Source: CAD feature listing. Evaluate the final solid. Frame: model axes, mm. Face numbers are marked on the shaded views. A direction names the side the tool comes from. Round coordinates to 2 decimals unless told otherwise and drop trailing zeros. Order: outer loops, then holes, each group sorted by start corner. A loop starts at its lowest first (then second) coordinate and runs counter-clockwise, first axis right, second up. Notation, with made-up numbers: (14.5, 48) -> (34.5, 48) arc R21 ccw to (34.5, 87) -> close; hole circle Ø4 at (65, -31). An arc over 180 degrees is marked (long way). One line per item, written item: value. Start each with the question number.
1) Ray query, L1, parallel to Z at x = -440, y = 591.25; L2, parallel to X at y = 587, z = -327; L3, parallel to X at y = 386, z = -241.5. Return the intervals inside material, ascending.
2) Reachability of the marked faces 1 and 2 from +Z, -Z, +X, -X, +Y, -Y: full face, straight path, thin tool, end or side. Return the list, or none.
3) Mould query, pull axis X, two halves, no side actions, for the marked faces 3, 4 and 5. Classes: pulls with the +X half, pulls with the -X half, needs draft (parallel to the pull), parting line crosses it, or undercut.
4) Section C-C (x = 178). Return the cut outline in (y, z).
5) Pin query (flat end, axial travel): P1, Ø7, axis at x = -440, z = -327.5, coming from the +Y side; P2, Ø13, axis at x = 440, z = -327.5, coming from the +Y side. Return the tip coordinate at first contact, or that it passes through.
6) Section B-B (z = 249.5). Return the cut outline in (x, y), and give its area (3 significant figures).
7) Section A-A (y = 87.5). Return the cut outline in (x, z), and give its area (3 significant figures).
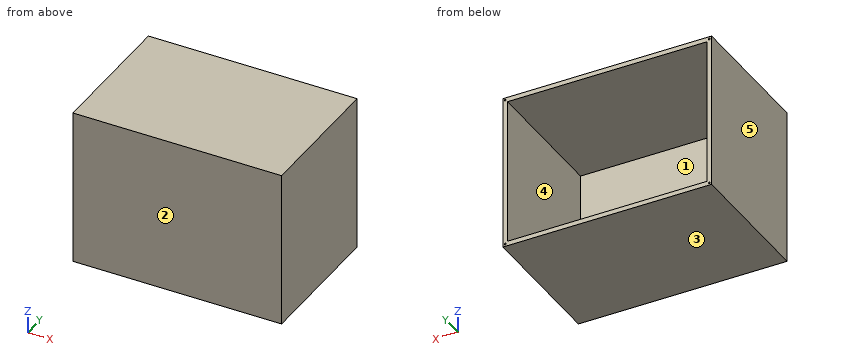
```python
from build123d import *

# Parameters (mm, degrees)
SKETCH1_W           = 900
SKETCH1_H           = 675
BOSS_EXTRUDE1_DEPTH = 600
SHELL1_T            = -20
SKETCH5_R           = 4
CUT_EXTRUDE1_DEPTH  = 20
SKETCH6_R           = 4
CUT_EXTRUDE2_DEPTH  = 20
SKETCH7_R           = 4
CUT_EXTRUDE3_DEPTH  = 20
SKETCH8_R           = 4
CUT_EXTRUDE4_DEPTH  = 20


with BuildPart() as part:
    # Sketch1 → Boss-Extrude1 (new body)
    with BuildSketch(Plane(origin=(0, 0, 0), x_dir=(1, 0, 0), z_dir=(0, 1, 0))):
        Rectangle(SKETCH1_W, SKETCH1_H)
    extrude(amount=BOSS_EXTRUDE1_DEPTH)

    # Shell1
    shell1_openings = [part.faces().sort_by_distance(p)[0] for p in [
        (0, 600, 0),
    ]]
    offset(amount=SHELL1_T, openings=shell1_openings, kind=Kind.INTERSECTION)

    # Sketch5 → Cut-Extrude1 (cut)
    with BuildSketch(Plane(origin=(0, 600, 0), x_dir=(1, 0, 0), z_dir=(0, 1, 0))):
        with Locations(Location((-440, -327.5, 0), (0, 0, 270))):
            Circle(SKETCH5_R)
    extrude(amount=-CUT_EXTRUDE1_DEPTH, mode=Mode.SUBTRACT)

    # Sketch6 → Cut-Extrude2 (cut)
    with BuildSketch(Plane(origin=(0, 600, 0), x_dir=(1, 0, 0), z_dir=(0, 1, 0))):
        with Locations(Location((440, -327.5, 0), (0, 0, 270))):
            Circle(SKETCH6_R)
    extrude(amount=-CUT_EXTRUDE2_DEPTH, mode=Mode.SUBTRACT)

    # Sketch7 → Cut-Extrude3 (cut)
    with BuildSketch(Plane(origin=(0, 600, 0), x_dir=(1, 0, 0), z_dir=(0, 1, 0))):
        with Locations(Location((440, 327.5, 0), (0, 0, 270))):
            Circle(SKETCH7_R)
    extrude(amount=-CUT_EXTRUDE3_DEPTH, mode=Mode.SUBTRACT)

    # Sketch8 → Cut-Extrude4 (cut)
    with BuildSketch(Plane(origin=(0, 600, 0), x_dir=(1, 0, 0), z_dir=(0, 1, 0))):
        with Locations(Location((-440, 327.5, 0), (0, 0, 270))):
            Circle(SKETCH8_R)
    extrude(amount=-CUT_EXTRUDE4_DEPTH, mode=Mode.SUBTRACT)


solid = part.part
```
Findings:
1. L1: -337.5 to -331.5, -323.5 to 323.5, 331.5 to 337.5
1. L2: -450 to -443.97, -436.03 to 436.03, 443.97 to 450
1. L3: -450 to -430, 430 to 450
2. face 1: +Y
2. face 2: +Z, -Z, +X, -X, -Y
3. face 3: needs draft
3. face 4: undercut
3. face 5: pulls with the -X half
4. outline: (0, -337.5) -> (600, -337.5) -> (600, -317.5) -> (20, -317.5) -> (20, 317.5) -> (600, 317.5) -> (600, 337.5) -> (0, 337.5) -> close
5. P1: y = 580
5. P2: y = 600
6. outline: (-450, 0) -> (450, 0) -> (450, 600) -> (430, 600) -> (430, 20) -> (-430, 20) -> (-430, 600) -> (-450, 600) -> close
6. area: 41,200 mm2
7. outline: (-450, -337.5) -> (450, -337.5) -> (450, 337.5) -> (-450, 337.5) -> close; hole (-430, -317.5) -> (430, -317.5) -> (430, 317.5) -> (-430, 317.5) -> close
7. area: 61,400 mm2
